from build123d import *

# Parameters (mm, degrees)
SKETCH_1_W      = 50
SKETCH_1_H      = 20
SKETCH_1_R      = 2.5
EXTRUDE_1_DEPTH = 2
SKETCH_1_3_R    = 2.5
EXTRUDE_2_DEPTH = 7


with BuildPart() as part:
    # Sketch 1 → Extrude 1 (new body)
    with BuildSketch(Plane(origin=(0, 0, 0), x_dir=(1, 0, 0), z_dir=(0, 1, 0))):
        Rectangle(SKETCH_1_W, SKETCH_1_H)
        with Locations(Location((-18, 3.8, 0), (0, 0, 270))):
            Circle(SKETCH_1_R, mode=Mode.SUBTRACT)
        with Locations(Location((-18, -3.8, 0), (0, 0, 90))):
            Circle(SKETCH_1_R, mode=Mode.SUBTRACT)
    extrude(amount=EXTRUDE_1_DEPTH)

    # Sketch 1_3 → Extrude 2 (add)
    with BuildSketch(Plane(origin=(0, 0, 0), x_dir=(1, 0, 0), z_dir=(0, 1, 0))):
        with Locations(Location((-18, 3.8, 0), (0, 0, 270))):
            Circle(SKETCH_1_3_R)
        with Locations(Location((-18, -3.8, 0), (0, 0, 270))):
            Circle(SKETCH_1_3_R)
    extrude(amount=EXTRUDE_2_DEPTH)


solid = part.part
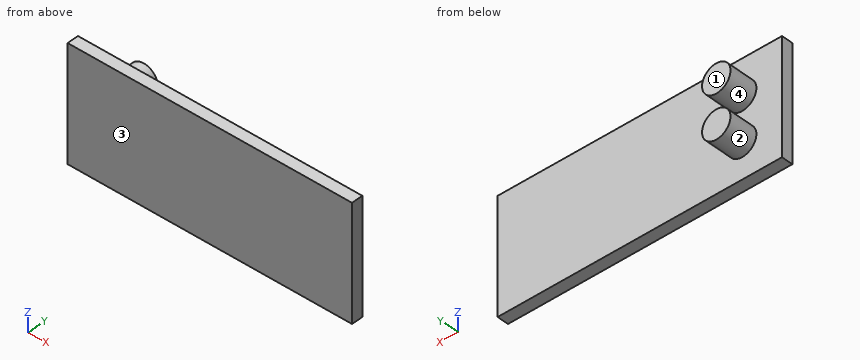
Verification items for the finished model (mm, model axes). Face numbers are marked on the shaded views. A direction names the side the tool comes from. Coordinates: 2 decimals unless noted, no trailing zeros. Order: outer loops, then holes, each group sorted by start corner. A loop starts at its lowest first (then second) coordinate and runs counter-clockwise, first axis right, second up. Notation, with made-up numbers: M 14.5,85.5 L 30.5,85.5 A19 cw 30.5,114.5 Z; hole C 25,86 d5. An arc over 180 degrees is marked long. One line per item, written item: value. Start each with the question number.
Item 1: Sectioned sample at A-A (x = -18). Enter the section's corners in (y, z), then the cut area to 3 significant figures.
Item 2: Sectioned sample at C-C (y = 6.25). Enter the section's corners in (x, z), then the cut area to 3 significant figures.
Item 3: Gauge pin test, flat ends, axial feed: pin 1 (6 mm diameter, centred on x = -10, z = 1, fed in from +Y); pin 2 (1.5 mm diameter, centred on x = 20, y = 3, fed in from +Z). Record the tip position at first contact, or that the pin passes through.
Item 4: Mould release check, pull along Z, two halves, no side actions. Record for the marked faces 3 and 4: released by +Z, released by -Z, zero draft, split by the parting line, or undercut.
Item 5: Access from +Z, -Z, +X, -X, +Y, -Y to the whole of each face (thin tool, end or side, straight path). Record for the marked faces 1 and 2.
Item 6: Scan lines: probe 1 along Y at (x, z) = (13.5, -3); probe 2 along X at (y, z) = (4, -3.25); probe 3 along X at (y, z) = (3, -5). Record each from-to range of solid material in increasing order.
Item 7: Sectioned sample at D-D (x = 2). Enter the section's corners in (y, z).
Item 8: Sectioned sample at B-B (z = 3.8). Enter the section's corners in (x, y), then the cut area to 3 significant figures.
Conclusion:
1. outline: M 0,-10 L 2,-10 L 2,-6.3 L 7,-6.3 L 7,-1.3 L 2,-1.3 L 2,1.3 L 7,1.3 L 7,6.3 L 2,6.3 L 2,10 L 0,10 Z
1. area: 90.0 mm^2
2. outline: C -18,-3.8 d5; C -18,3.8 d5
2. area: 39.3 mm^2
3. pin 1: stops at y = 2
3. pin 2: passes through
4. face 3: zero draft
4. face 4: undercut
5. face 1: +Z, -Z, +X, -X, +Y
5. face 2: +Y
6. probe 1: y = 0 to 2
6. probe 2: x = -20.44 to -15.56
6. probe 3: x = -20.19 to -15.81
7. outline: M 0,-10 L 2,-10 L 2,10 L 0,10 Z
8. outline: M -25,0 L 25,0 L 25,2 L -15.5,2 L -15.5,7 L -20.5,7 L -20.5,2 L -25,2 Z
8. area: 125 mm^2
